Can you work these out from the drawing? Everything is in mm from the part's minimum corner. Give positions to 0.01 mm unless a question says otherwise; leave off trailing zeros. Loops run counter-clockwise (first coordinate to the right, second up) from the corner with the lowest first, then second, coordinate; pieces in that order, holes last. Notation, with made-up numbers: (66.5, -24) - (120.5, -24) arc R19 ccw to (120.5, -12) - close; hole circle Ø10 at (82.25, -19). An arc over 180 degrees is marked (long way). Write each question's results on one line, items separated by ' | '. Start each with the question number.
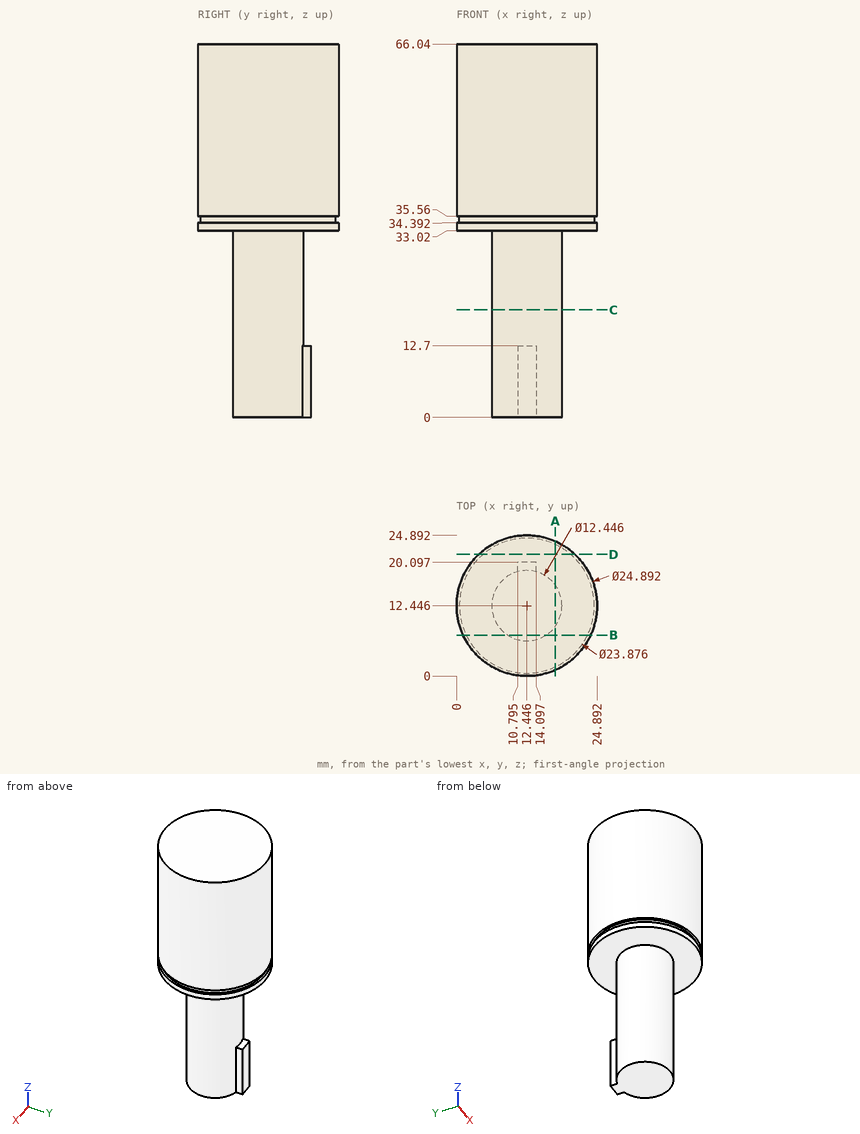
Q1. I want a section at C-C, the plane z = 19. List the corners of the cut face in (x, y) for me, then the cut area to 3 significant figures.
Q2. I want a section at B-B, the plane y = 7.25. List the corners of the cut face in (x, z) for me (1 decimal), then the cut area to 3 significant figures.
Q3. I want a section at D-D, the plane y = 21.5. List the corners of the cut face in (x, z) for me (1 decimal).
Q4. I'm going to push flat-ended pins straight in: pin 1 Ø1.8 at (y, z) = (19, 6.5) entering from -X (1 decimal); pin 2 Ø2 at (y, z) = (4, 7) entering from +X; pin 3 Ø8 at (x, z) = (19, 25.5) entering from +Y; pin 4 Ø6 at (y, z) = (10, 6.5) entering from -X. Where does each tip first touch, or does it pass through?
Q5. I need wall thicknesses on L1, parallel to Z at x = 23, y = 17.75; L2, parallel to X at y = 16.5, z = 14 (1 decimal); L3, parallel to Y at x = 16.75, z = 51 (1 decimal). Which ranges of each line are inside material? Lowest first, please. Write a range as from..to.
Q6. I want a section at A-A, the plane x = 17.5. List the corners of the cut face in (y, z) for me (1 decimal).
Conclusion:
1) outline: circle Ø12.45 at (12.45, 12.45) | area: 122 mm^2
2) outline: (1.1, 33) - (9, 33) - (9, 0) - (15.9, 0) - (15.9, 33) - (23.8, 33) - (23.8, 34.4) - (23.2, 34.4) - (23.2, 35.6) - (23.8, 35.6) - (23.8, 66) - (1.1, 66) - (1.1, 35.6) - (1.7, 35.6) - (1.7, 34.4) - (1.1, 34.4) - close | area: 972 mm^2
3) outline: (3.9, 33) - (21, 33) - (21, 34.4) - (20.2, 34.4) - (20.2, 35.6) - (21, 35.6) - (21, 66) - (3.9, 66) - (3.9, 35.6) - (4.7, 35.6) - (4.7, 34.4) - (3.9, 34.4) - close
4) pin 1: x = 9.8 | pin 2: through | pin 3: y = 18.12 | pin 4: x = 6.22
5) L1: 33.02..66.04 | L2: 7.7..17.2 | L3: 0.8..24.1
6) outline: (1.1, 33) - (8.8, 33) - (8.8, 0) - (16.1, 0) - (16.1, 33) - (23.8, 33) - (23.8, 34.4) - (23.3, 34.4) - (23.3, 35.6) - (23.8, 35.6) - (23.8, 66) - (1.1, 66) - (1.1, 35.6) - (1.6, 35.6) - (1.6, 34.4) - (1.1, 34.4) - close
